Autodesk Inventor part; units mm, degrees
ref_plane "YZ Plane" through (0, 0, 0) normal (1, 0, 0) x (0, 1, 0)
ref_plane "XZ Plane" through (0, 0, 0) normal (0, 1, 0) x (-1, 0, 0)
ref_plane "XY Plane" through (0, 0, 0) normal (0, 0, 1) x (1, 0, 0)
sketch "Эскиз3" plane through (0, 0, 0) normal (0, 0, 1) x (1, 0, 0)
  line L0 (-1.4, 0) -> (-1.4, -16)
  line L1 (-1.4, -16) -> (0, -16)
  line L2 (0, -16) -> (0, 2)
  line L3 (-1.4, 0) -> (-2.5, 0)
  arc A0 (-2.5, 2) -> (-2.5, 0) centre (-1.4, 1) ccw
  line L4 (-1.3, 2) -> (-0.5, 0.4)
  line L5 (-0.5, 0.4) -> (0, 0.4)
  line L6 (-2.5, 2) -> (-1.3, 2)
  point P0 (0, 0)
  dimension "d4" = 2.8
  dimension "d6" = 1
  dimension "d7" = 5
  dimension "d8" = 16
  dimension "d10" = 2
  dimension "d12" = 2.6
  dimension "d13" = 0.4
  dimension "d14" = 1
revolve "Вращение1" add sketch "Эскиз3" angle 360 about axis through (0, -16, 0) along (0, 1, 0)
sketch "Эскиз5" plane through (0, 0, 0) normal (0, 0, 1) x (1, 0, 0)
  line L0 (0.5, 0.4) -> (-0.5, 0.4)
  line L1 (-0.5, 0.4) -> (-2.2, 2)
  line L2 (2.5, 2) -> (-2.5, 2)
  line L3 (-2.2, 2) -> (0, 2)
  line L4 (1.3, 2) -> (-1.3, 2)
  line L5 (0, 0.4) -> (-0.5, 0.4)
  line L6 (0, 0.4) -> (0, 2)
  point P0 (0, 0)
  dimension "d15" = 2.2
extrude "Выдавливание2" cut sketch "Эскиз5" along normal mid plane 1
pattern_circular "Круговой массив1" count 4 over 360 about axis through (0, -10, 0) along (0, 1, 0) of "Выдавливание2"
thread "Резьба1"
properties part number "M3x16" material "Сталь, литейная"
The listing builds one solid part. Answer for the finished solid, in the listing's coordinates (mm). A direction names the side the tool comes from. Give positions to 0.01 mm unless a question says otherwise; leave off trailing zeros. Order: outer loops, then holes, each group sorted by start corner. A loop starts at its lowest first (then second) coordinate and runs counter-clockwise, first axis right, second up. Notation, with made-up numbers: M 87.5,-11 L 117.5,-11 A7 cw 117.5,-4 Z; hole C 35.5,43.5 d11. An arc over 180 degrees is marked long. Put each result on its own line as item: value. Start each with the question number.
Item 1: The part is cut by section A-A, the plane y = -13. Determine the outline of the cut face in (x, z), and give its area (3 significant figures).
Item 2: Find the intervals of material crossed by line 1 along Y through (x, z) = (-1.1, 1.25); line 2 along Z through (x, y) = (-0.1, -7.75); line 3 along X through (y, z) = (1, -0.7), in increasing order.
Item 3: For a pull along Z with two mould halves and no side action, classify faces 3 (the face through (1.4, -8.11, -0.06)), 4 (the face through (-1.1, 0, -1.1)), 5 (the face through (-0.5, 1.4, -1.2)) as +Z half, -Z half, draft (parallel to the pull), parting line (faces both ways), or undercut.
Item 4: Which of the six approach directions +Z, -Z, +X, -X, +Y, -Y give full straight-line access (tool end or side, diameter ignored) to faces 1 (the face through (0, -16, 0)), 2 (the face through (-1.2, 1.4, -0.5))?
Item 5: Flat-ended cylindrical pins translate along their axes: P1, Ø0.5, axis at x = 1.5, y = 1.5, coming from the -Z side; P2, Ø1.8, axis at y = 1, z = 1.5, coming from the +X side; P3, Ø1, axis at x = 1.5, y = -2, coming from the -Z side. Find the tip coordinate at first contact, or state that the pin passes through.
Answer key:
1. outline: C 0,0 d2.8
1. area: 6.16 mm²
2. line 1: y = 0 to 2
2. line 2: z = -1.4 to 1.4
2. line 3: x = -2.8 to -0.5, 0.5 to 2.8
3. face 3: parting line
3. face 4: draft
3. face 5: undercut
4. face 1: +Z, -Z, +X, -X, -Y
4. face 2: +Y
5. P1: stops at z = -2.53
5. P2: stops at x = 2.82
5. P3: stops at z = -0.98
